Here's the drawing with two shaded views (mm, measured from the low corner). I have some questions. Give positions to 0.01 mm unless a question says otherwise; leave off trailing zeros. Write each loop counter-clockwise with the first axis right and the second up, starting at its lowest first coordinate (ties: lowest second). Pieces come first, ordered by that corner, then holes.
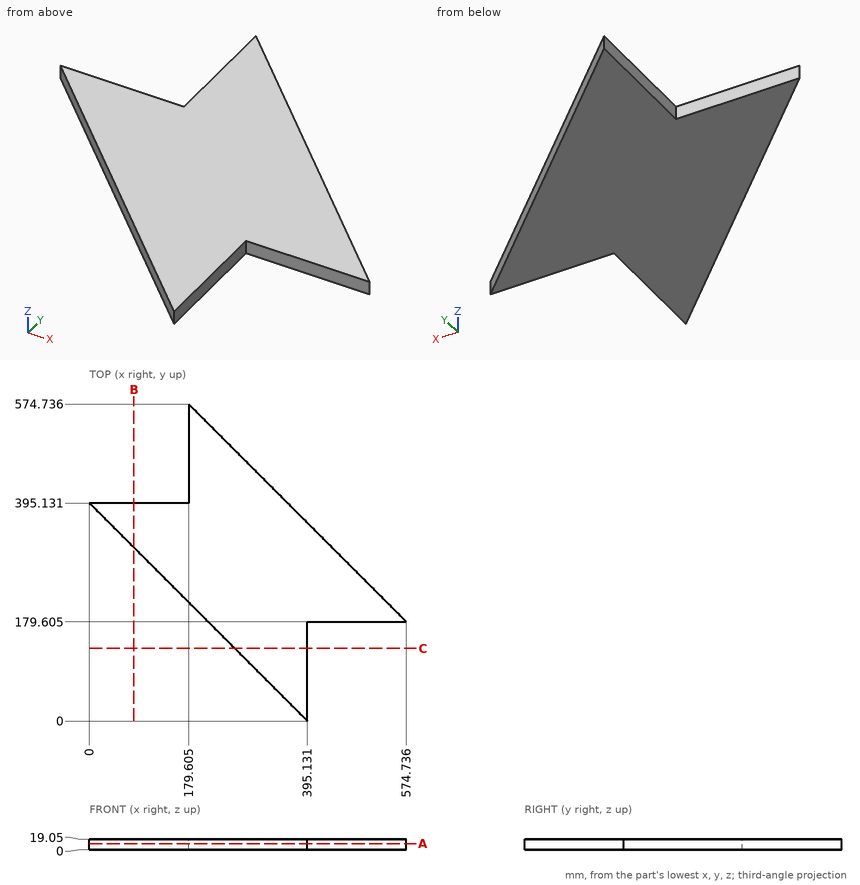
(1) Imagine slicing it at C-C, the plane y = 131.5. Write out the boundary of the cut face in (x, z), plus the area to 4 significant figures.
Returned:
outline: (263.63, 0) - (395.13, 0) - (395.13, 19.05) - (263.63, 19.05) - close
area: 2,505 mm2
(2) Will these pins go through, and if not, where does the flat tip stop? P1, Ø10, axis at x = 216, z = 12, coming from the -Y side; P2, Ø8, axis at x = 466, z = 14, coming from the +Y side; P3, Ø10, axis at y = 314.5, z = 7, coming from the +X side.
Returned:
P1: stops at y = 174.13
P2: stops at y = 292.34
P3: stops at x = 444.84
(3) Imagine slicing it at B-B, the plane x = 80.5. Write out the boundary of the cut face in (y, z), plus the area to 3 significant figures.
Returned:
outline: (314.63, 0) - (395.13, 0) - (395.13, 19.05) - (314.63, 19.05) - close
area: 1,530 mm2
(4) Imagine slicing it at A-A, the plane z = 10.5. Write out the boundary of the cut face in (x, y) (1 decimal), plus the area to 3 significant figures.
Returned:
outline: (0, 395.1) - (395.1, 0) - (395.1, 179.6) - (574.7, 179.6) - (179.6, 574.7) - (179.6, 395.1) - close
area: 110,000 mm2
(5) If I drill on L1, parallel to Y at x = 174, z = 6.25; L2, parallel to X at y = 105.5, z = 15; L3, parallel to X at y = 250.5, z = 10.75, over which ranges is the centre line in solid material (lowest first)?
Returned:
L1: y = 221.13 to 395.13
L2: x = 289.63 to 395.13
L3: x = 144.63 to 503.84
